The figure shows three views and two pictorial views of one solid part (mm, origin at its lowest corner). Answer the questions. Coordinates: 2 decimals unless noted, no trailing zeros. Write each loop counter-clockwise with the first axis right and the second up, starting at its lowest first coordinate (ties: lowest second). Pieces come first, ordered by that corner, then holes.
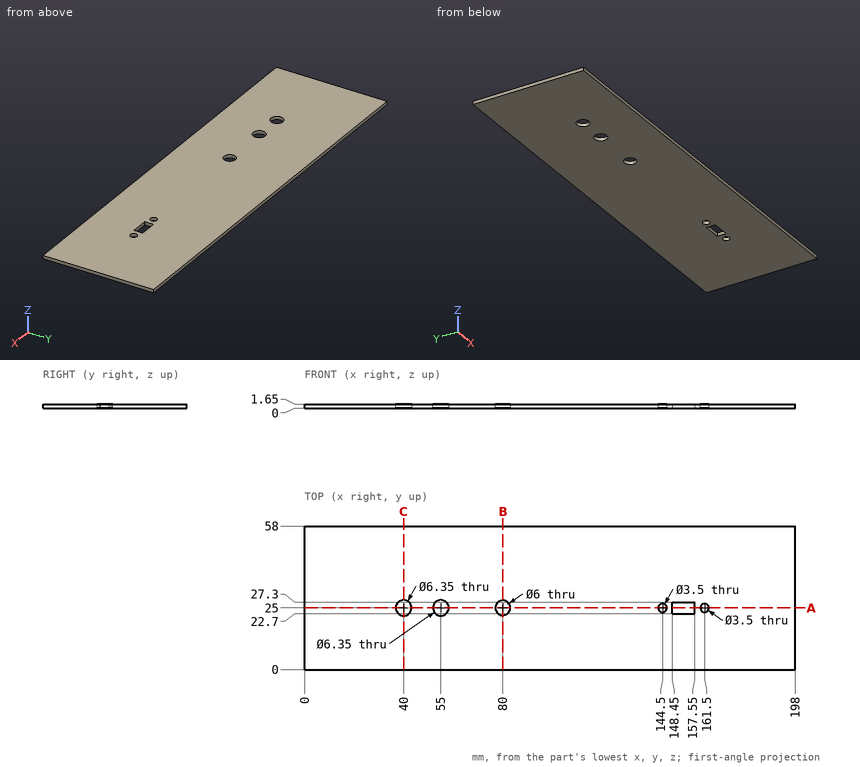
1. Section A-A on y = 25 is taken. Give the vertices of the cut face in (x, z) (3 decimals).
Results found:
outline: (0, 0) - (36.825, 0) - (36.825, 1.65) - (0, 1.65) - close; (43.175, 0) - (51.825, 0) - (51.825, 1.65) - (43.175, 1.65) - close; (58.175, 0) - (77, 0) - (77, 1.65) - (58.175, 1.65) - close; (83, 0) - (142.75, 0) - (142.75, 1.65) - (83, 1.65) - close; (146.25, 0) - (148.45, 0) - (148.45, 1.65) - (146.25, 1.65) - close; (157.55, 0) - (159.75, 0) - (159.75, 1.65) - (157.55, 1.65) - close; (163.25, 0) - (198, 0) - (198, 1.65) - (163.25, 1.65) - close
2. Section B-B on x = 80 is taken. Give the vertices of the cut face in (y, z).
Results found:
outline: (0, 0) - (22, 0) - (22, 1.65) - (0, 1.65) - close; (28, 0) - (58, 0) - (58, 1.65) - (28, 1.65) - close
3. Section C-C on x = 40 is taken. Give the vertices of the cut face in (y, z) (3 decimals), then the cut area to 3 significant figures.
Results found:
outline: (0, 0) - (21.825, 0) - (21.825, 1.65) - (0, 1.65) - close; (28.175, 0) - (58, 0) - (58, 1.65) - (28.175, 1.65) - close
area: 85.2 mm2
4. A flat-ended cylindrical pin translates along its axis: P1, Ø3, axis at x = 144.5, y = 25, coming from the -Z side. Find the tip coordinate at first contact, or state that the pin passes through.
Results found:
P1: passes through
5. Find the intervals of material crossed by L1, parallel to Y at x = 55, z = 1.1 (3 decimals); L2, parallel to Y at x = 39, z = 1, in increasing order.
Results found:
L1: y = 0 to 21.825, 28.175 to 58
L2: y = 0 to 21.99, 28.01 to 58
